from build123d import *

# Parameters (mm, degrees)
SKETCH1_W               = 3
SKETCH1_H               = 12
SKETCH1_H_2             = 18
BOSS_EXTRUDE1_DEPTH     = 3.175
SKETCH2_W               = 32.65
SKETCH2_H               = 2
BOSS_EXTRUDE2_DEPTH     = 3.175
CUT_EXTRUDE1_DEPTH      = 28.227031605
CUT_EXTRUDE1_DEPTH_BACK = 28.227031605
SKETCH3_W               = 3
SKETCH3_H               = 2


with BuildPart() as part:
    # Sketch1 → Boss-Extrude1 (new body)
    with BuildSketch(Plane.XY):
        Polygon((19.825, 5.331730769), (-19.825, 12.5), (-19.825, 10), (-19.825, -8), (-19.825, -12.5), (19.825, -12.5), (19.825, -8), (19.825, 4), align=None)
        with Locations((21.325, -2)):
            Rectangle(SKETCH1_W, SKETCH1_H)
        with Locations((-21.325, 1)):
            Rectangle(SKETCH1_W, SKETCH1_H_2)
    extrude(amount=BOSS_EXTRUDE1_DEPTH)

    # Sketch2 → Boss-Extrude2 (add)
    with BuildSketch(Plane.XY.offset(3.175)):
        with Locations((3.5, -13.5)):
            Rectangle(SKETCH2_W, SKETCH2_H)
    extrude(amount=-BOSS_EXTRUDE2_DEPTH)

    # Sketch3 → Cut-Extrude1 (cut, two sides: drawn at the far end of the back side and taken through both)
    with BuildSketch(Plane.XY.offset(3.175).offset(-CUT_EXTRUDE1_DEPTH_BACK)):
        with Locations((-21.325, 0.5)):
            Rectangle(SKETCH3_W, SKETCH3_H)
    extrude(amount=CUT_EXTRUDE1_DEPTH + CUT_EXTRUDE1_DEPTH_BACK, mode=Mode.SUBTRACT)


solid = part.part
Verification items for the finished model (mm, model axes). A direction names the side the tool comes from. Coordinates: 2 decimals unless noted, no trailing zeros. Order: outer loops, then holes, each group sorted by start corner. A loop starts at its lowest first (then second) coordinate and runs counter-clockwise, first axis right, second up.
Item 1: Release check for a two-part mould opening along Y. For faces 4 (the face through (21, 4, 2)), 5 (the face through (-12.825, -14, 2)), 6 (the face through (-21, 1.5, 2)) record: +Y half, -Y half, draft (parallel to the pull), parting line (faces both ways), or undercut.
Filled in:
face 4: +Y half
face 5: draft
face 6: undercut
Item 2: Material ranges on L1, parallel to X at y = -11, z = 1.45 (3 decimals); L2, parallel to Y at x = 20, z = 3; L3, parallel to Y at x = -4.5, z = 2.6, recorded low to high.
Filled in:
L1: x = -19.825 to 19.825
L2: y = -8 to 4
L3: y = -14.5 to 9.73
Item 3: Section check B-B, the plane y = 4.75. Enter the section's corners in (x, z) (3 decimals), then the cut area to 3 significant figures.
Filled in:
outline: (-22.825, 0) - (19.825, 0) - (19.825, 3.175) - (-22.825, 3.175) - close
area: 135 mm2
Item 4: Depth check by flat-ended pin: pin 1 (1.5 mm diameter, centred on x = -20.5, z = 2.5, fed in from -Y); pin 2 (0.6 mm diameter, centred on y = -13.5, z = 1, fed in from -X) (3 decimals); pin 3 (1.5 mm diameter, centred on x = -21, z = 2.5, fed in from -Y). Enter the tip coordinate at first touch or a pass-through.
Filled in:
pin 1: stops at y = -12.5
pin 2: stops at x = -12.825
pin 3: stops at y = -8
Item 5: Section check C-C, the plane x = -3. Enter the section's corners in (y, z) (3 decimals), then the cut area to 3 significant figures.
Filled in:
outline: (-14.5, 0) - (9.458, 0) - (9.458, 3.175) - (-14.5, 3.175) - close
area: 76.1 mm2
Item 6: Section check A-A, the plane z = 0.7. Enter the section's corners in (x, y) (3 decimals).
Filled in:
outline: (-22.825, -8) - (-19.825, -8) - (-19.825, -12.5) - (-12.825, -12.5) - (-12.825, -14.5) - (19.825, -14.5) - (19.825, -8) - (22.825, -8) - (22.825, 4) - (19.825, 4) - (19.825, 5.332) - (-19.825, 12.5) - (-19.825, 10) - (-22.825, 10) - (-22.825, 1.5) - (-19.825, 1.5) - (-19.825, -0.5) - (-22.825, -0.5) - close
Item 7: Access from +Z, -Z, +X, -X, +Y, -Y to the whole of each face (thin tool, end or side, straight path). Record for faces 1 (the face through (-19.825, 0, 2)), 2 (the face through (-19.825, 11, 2)), 3 (the face through (-16, -12.5, 2)).
Filled in:
face 1: +Z, -Z, -X
face 2: +Z, -Z, -X, +Y
face 3: +Z, -Z, -X, -Y
